Geometry check sheet. Reference: the model listing, model coordinates, mm. Coordinates: 2 decimals unless noted, no trailing zeros. Write each loop counter-clockwise with the first axis right and the second up, starting at its lowest first coordinate (ties: lowest second). Pieces come first, ordered by that corner, then holes. Notation, with made-up numbers: (-5, 9) -> (4, 9) arc R19 ccw to (4, 34) -> close; hole circle Ø11 at (0.25, 24). An arc over 180 degrees is marked (long way). One line per question, with ' | ' between items.
from build123d import *

# Parameters (mm, degrees)
SKETCH1_R               = 11.1
SKETCH1_R_2             = 8.1
BOSS_EXTRUDE1_DEPTH     = 50
SKETCH3_W               = 203.170281232
SKETCH3_H               = 205.602397066
CUT_EXTRUDE1_DEPTH      = 53.406297332
SKETCH4_R               = 11.1
BOSS_EXTRUDE3_DEPTH     = 3
CUT_EXTRUDE2_DEPTH      = 99.261996723
CUT_EXTRUDE2_DEPTH_BACK = 99.261996723
SKETCH5_R               = 2.6
SKETCH6_W               = 15
SKETCH6_H               = 30
BOSS_EXTRUDE4_DEPTH     = 1.5
CUT_EXTRUDE3_DEPTH      = 60.691875494
CUT_EXTRUDE3_DEPTH_BACK = 60.691875494
SKETCH7_W               = 115.313009773
SKETCH7_H               = 104.745429411
BOSS_EXTRUDE5_START     = -8
SKETCH8_R               = 14.1
SKETCH8_R_2             = 11.1
BOSS_EXTRUDE5_DEPTH     = 8
FILLET3_R               = 1.5


with BuildPart() as part:
    # Sketch1 → Boss-Extrude1 (new, symmetric)
    with BuildSketch(Plane(origin=(0, 0, 0), x_dir=(1, 0, 0), z_dir=(0, 1, 0))):
        with Locations(Location((0, 0, 0), (0, 0, 270))):
            Circle(SKETCH1_R)
        with Locations(Location((0, 0, 0), (0, 0, 270))):
            Circle(SKETCH1_R_2, mode=Mode.SUBTRACT)
    extrude(amount=BOSS_EXTRUDE1_DEPTH, both=True)

    # Sketch3 → Cut-Extrude1 (cut, through all)
    with BuildSketch(Plane.XY):
        Rectangle(SKETCH3_W, SKETCH3_H)
    extrude(amount=CUT_EXTRUDE1_DEPTH, mode=Mode.SUBTRACT)

    # Sketch4 → Boss-Extrude3 (add, symmetric)
    with BuildSketch(Plane.XZ.offset(50)):
        with Locations(Location((0, 0, 0), (0, 0, 270))):
            Circle(SKETCH4_R)
    extrude(amount=BOSS_EXTRUDE3_DEPTH, both=True)

    # Sketch5 → Cut-Extrude2 (cut, two sides: drawn at the far end of the back side and taken through both)
    with BuildSketch(Plane(origin=(0, -47, 0), x_dir=(1, 0, 0), z_dir=(0, 1, 0)).offset(-CUT_EXTRUDE2_DEPTH_BACK)):
        with Locations(Location((0, 0, 0), (0, 0, 270))):
            Circle(SKETCH5_R)
    extrude(amount=CUT_EXTRUDE2_DEPTH + CUT_EXTRUDE2_DEPTH_BACK, mode=Mode.SUBTRACT)

    # Sketch6 → Boss-Extrude4 (add, symmetric)
    with BuildSketch(Plane.XY.offset(-6)):
        with Locations((15.1, 25)):
            Rectangle(SKETCH6_W, SKETCH6_H)
        with Locations((-15.1, 25)):
            Rectangle(SKETCH6_W, SKETCH6_H)
    extrude(amount=BOSS_EXTRUDE4_DEPTH, both=True)

    # Sketch7 → Cut-Extrude3 (cut, two sides: drawn at the far end of the back side and taken through both)
    with BuildSketch(Plane.XY.offset(-4.5).offset(-CUT_EXTRUDE3_DEPTH_BACK)):
        with Locations((3.022672806, 5.372714706)):
            Rectangle(SKETCH7_W, SKETCH7_H)
    extrude(amount=CUT_EXTRUDE3_DEPTH + CUT_EXTRUDE3_DEPTH_BACK, mode=Mode.SUBTRACT)

    # Sketch8 → Boss-Extrude5 (add)
    with BuildSketch(Plane.XZ.offset(53).offset(BOSS_EXTRUDE5_START)):
        with Locations(Location((0, 0, 0), (0, 0, 270))):
            Circle(SKETCH8_R)
        with Locations(Location((0, 0, 0), (0, 0, 270))):
            Circle(SKETCH8_R_2, mode=Mode.SUBTRACT)
    extrude(amount=BOSS_EXTRUDE5_DEPTH)

    # Fillet3
    fillet3_edges = [part.edges().sort_by_distance(p)[0] for p in [
        (0, -45, 14.1),
        (0, -45, 11.1),
    ]]
    fillet(fillet3_edges, radius=FILLET3_R - 0.0001)  # a hair under: the kernel refuses the full size


solid = part.part
1. Mould release check, pull along Z, two halves, no side actions. Record for faces 1 (the face through (0.78, -50.04, 2.48)), 2 (the face through (0, -53, -3)), 3 (the face through (-5.4, -49.704, -13.025)): released by +Z, released by -Z, zero draft, split by the parting line, or undercut.
Worked answers:
face 1: undercut | face 2: zero draft | face 3: split by the parting line
2. Material ranges on line 1 (X direction, y = -46.75, z = 0); line 2 (X direction, y = -48.7, z = 0); line 3 (Y direction, x = 4, z = 9.75), recorded low to high. Write a range as from..to.
Worked answers:
line 1: -14.1..-11.1, 11.1..14.1 | line 2: -14.1..-2.6, 2.6..14.1 | line 3: -53..-47
3. Go/stop test with flat-tipped pins: P1, Ø6.5, axis at x = 1.5, z = 2.5, coming from the +Y side; P2, Ø3, axis at x = 9, y = -46.5, coming from the -Z side; P3, Ø4, axis at x = -9, y = -49, coming from the -Z side. Record where each tip stops, or that it passes through.
Worked answers:
P1: y = -47 | P2: z = -11.94 | P3: z = -12.24
4. Cross-section at C-C on y = -49. Record the boundary of the cut face in (x, z).
Worked answers:
outline: circle Ø28.2 at (0, 0); hole circle Ø5.2 at (0, 0)
